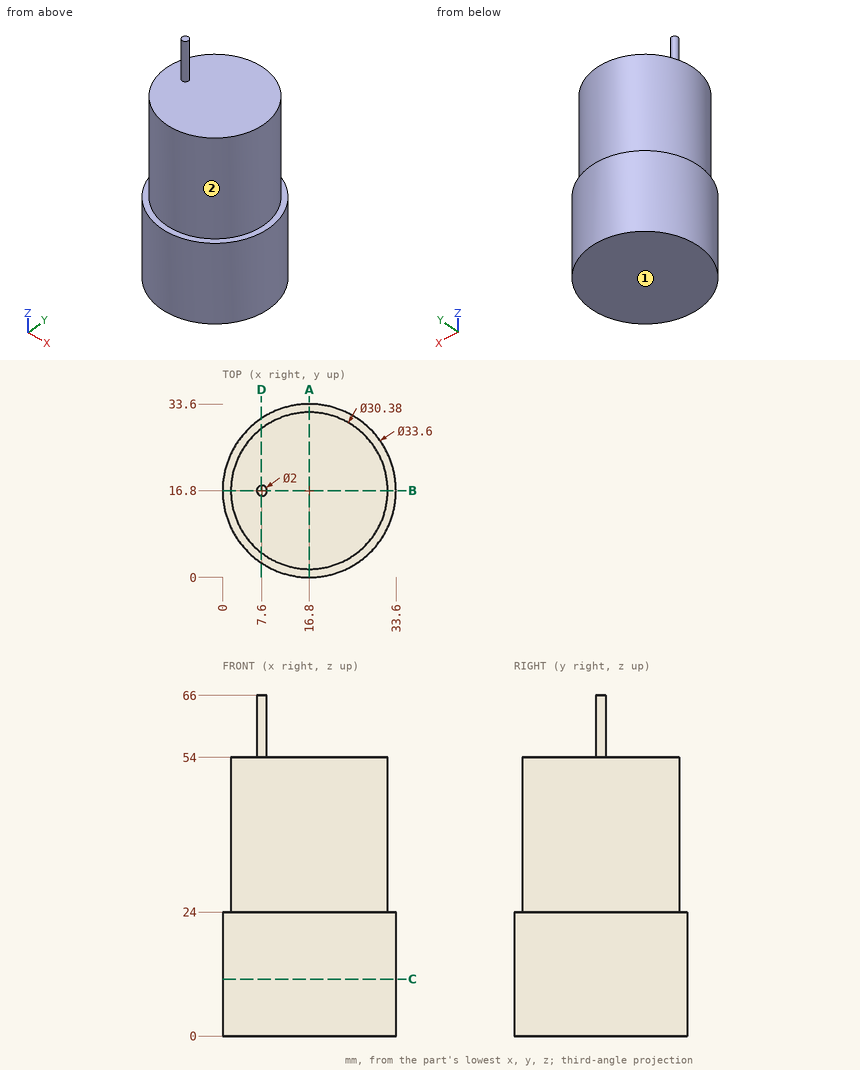
Source: three-view drawing plus pictorial views. Frame: mm from the lowest corner of the part. A direction names the side the tool comes from. Coordinates: 2 decimals unless noted, no trailing zeros. Order: outer loops, then holes, each group sorted by start corner. A loop starts at its lowest first (then second) coordinate and runs counter-clockwise, first axis right, second up. Notation, with made-up numbers: M 46,43.5 L 54,43.5 A19 cw 54,65.5 Z; hole C 24.25,45 d7. An arc over 180 degrees is marked long. Write each question's results on one line, items separated by ' | '. Start each with the question number.
1. Material intervals for L1, parallel to Z at x = 10, y = 19.5; L2, parallel to Z at x = 12, y = 31.5; L3, parallel to X at y = 21, z = 40.5, sorted ascending.
2. Pin query (flat end, axial travel): pin 1 (10 mm diameter, centred on y = 8.5, z = 18, fed in from -X); pin 2 (10 mm diameter, centred on y = 30, z = 44, fed in from +X); pin 3 (3 mm diameter, centred on y = 11.5, z = 36, fed in from +X). Return the tip coordinate at first contact, or that it passes through.
3. Section D-D, the plane x = 7.5. Return the cut outline in (y, z).
4. Reachability of the marked faces 1 and 2 from +Z, -Z, +X, -X, +Y, -Y: full face, straight path, thin tool, end or side. Return the list, or none.
5. Section A-A, the plane x = 16.8. Return the cut outline in (y, z), then the cut area to 3 significant figures.
6. Section B-B, the plane y = 16.8. Return the cut outline in (x, z), then the cut area to 3 significant figures.
7. Section C-C, the plane z = 11. Return the cut outline in (x, y), then the cut area to 3 significant figures.
Solution:
1) L1: 0 to 54 | L2: 0 to 24 | L3: 2.2 to 31.4
2) pin 1: x = 0.33 | pin 2: x = 29.59 | pin 3: x = 31.51
3) outline: M 2.81,0 L 30.79,0 L 30.79,24 L 28.81,24 L 28.81,54 L 17.79,54 L 17.79,66 L 15.81,66 L 15.81,54 L 4.79,54 L 4.79,24 L 2.81,24 Z
4) face 1: -Z, +X, -X, +Y, -Y | face 2: +Z
5) outline: M 0,0 L 33.6,0 L 33.6,24 L 31.99,24 L 31.99,54 L 1.61,54 L 1.61,24 L 0,24 Z | area: 1,720 mm²
6) outline: M 0,0 L 33.6,0 L 33.6,24 L 31.99,24 L 31.99,54 L 8.6,54 L 8.6,66 L 6.6,66 L 6.6,54 L 1.61,54 L 1.61,24 L 0,24 Z | area: 1,740 mm²
7) outline: C 16.8,16.8 d33.6 | area: 887 mm²
